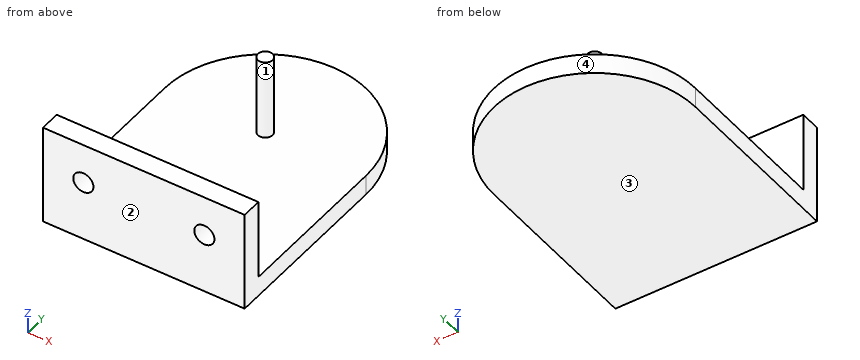
from build123d import *

# Parameters (mm, degrees)
BOSS_EXTRUDE1_DEPTH = 3.175
SKETCH4_W           = 31.75
SKETCH4_H           = 3.175
BOSS_EXTRUDE2_DEPTH = 12.7
SKETCH5_R           = 1.5875
CUT_EXTRUDE2_DEPTH  = 47.651371748
SKETCH6_R           = 1.15
BOSS_EXTRUDE3_DEPTH = 12.7


with BuildPart() as part:
    # Sketch1 → Boss-Extrude1 (new body)
    with BuildSketch(Plane.XY):
        with BuildLine():
            ThreePointArc((15.875, 0), (0, 15.875), (-15.875, 0))
            Line((-15.875, 0), (15.875, 0))
        make_face()
        with BuildLine():
            ThreePointArc((15.875, 0), (0, -15.875), (-15.875, 0))
            Line((-15.875, 0), (-15.875, -28.194))
            Line((-15.875, -28.194), (15.875, -28.194))
            Line((15.875, -28.194), (15.875, 0))
        make_face()
        with BuildLine():
            Line((15.875, 0), (-15.875, 0))
            ThreePointArc((-15.875, 0), (0, -15.875), (15.875, 0))
        make_face()
    extrude(amount=BOSS_EXTRUDE1_DEPTH)

    # Sketch4 → Boss-Extrude2 (add)
    with BuildSketch(Plane.XY.offset(3.175)):
        with Locations((0, -26.6065)):
            Rectangle(SKETCH4_W, SKETCH4_H)
    extrude(amount=BOSS_EXTRUDE2_DEPTH)

    # Sketch5 → Cut-Extrude2 (cut, through all)
    with BuildSketch(Plane(origin=(0, -25.019, 0), x_dir=(1, 0, 0), z_dir=(0, 1, 0))):
        with Locations(Location((-9.525, -9.525, 0), (0, 0, 270))):
            Circle(SKETCH5_R)
        with Locations(Location((9.525, -9.525, 0), (0, 0, 90))):
            Circle(SKETCH5_R)
    extrude(amount=-CUT_EXTRUDE2_DEPTH, mode=Mode.SUBTRACT)

    # Sketch6 → Boss-Extrude3 (add, through all)
    with BuildSketch(Plane.XY.offset(3.175)):
        Circle(SKETCH6_R)
    extrude(amount=BOSS_EXTRUDE3_DEPTH)


solid = part.part
Can you work these out from the model? Positions are in its coordinate system, mm. Face numbers are marked on the shaded views. Give positions to 0.01 mm unless a question says otherwise; leave off trailing zeros. Loops run counter-clockwise (first coordinate to the right, second up) from the corner with the lowest first, then second, coordinate; pieces in that order, holes last. Notation, with made-up numbers: (-4, 7.5) - (7, 7.5) arc R19 ccw to (7, 32.5) - close; hole circle Ø3 at (57, 18.25). An arc over 180 degrees is marked (long way). Return JSON: item names as keys, results as strings.
1. I'm going to push flat-ended pins straight in: pin 1 Ø6 at (x, y) = (-6.5, -5.5) entering from +Z (3 decimals); pin 2 Ø8 at (x, z) = (12, 1.5) entering from +Y; pin 3 Ø6 at (x, z) = (-12, 2) entering from +Y; pin 4 Ø10 at (x, y) = (6, -4.5) entering from -Z. Where does each tip first touch, or does it pass through?
Output values:
{"pin 1": "stops at z = 3.175", "pin 2": "stops at y = 13.71", "pin 3": "stops at y = 13.08", "pin 4": "stops at z = 0"}
2. If I drill on line 1 (Z direction, x = 0.5, y = 8) (3 decimals); line 2 (Y direction, x = 0.5, z = 2.25); line 3 (Y direction, x = -5, z = 11), over which ranges is the centre line in solid material (lowest first)?
Output values:
{"line 1": "z = 0 to 3.175", "line 2": "y = -28.19 to 15.87", "line 3": "y = -28.19 to -25.02"}
3. We'd pull the mould along Y, two halves only. Please class the marked faces 1, 2, 3 and 4: +Y half, -Y half, draft (parallel to the pull), parting line (faces both ways), or undercut.
Output values:
{"face 1": "undercut", "face 2": "-Y half", "face 3": "draft", "face 4": "+Y half"}
4. I want a section at D-D on z = 2.5. Please give me the cut outline in (x, y) (3 decimals), and give its area (3 significant figures).
Output values:
{"outline": "(-15.875, -28.194) - (15.875, -28.194) - (15.875, 0) arc R15.875 ccw to (-15.875, 0) - close", "area": "1,290 mm²"}
5. I want a section at A-A on z = 12. Please give me the cut outline in (x, y) (3 decimals).
Output values:
{"outline": "(-15.875, -28.194) - (15.875, -28.194) - (15.875, -25.019) - (-15.875, -25.019) - close; circle Ø2.3 at (0, 0)"}
6. I want a section at B-B on x = 0. Please give me the cut outline in (y, z) (3 decimals).
Output values:
{"outline": "(-28.194, 0) - (15.875, 0) - (15.875, 3.175) - (1.15, 3.175) - (1.15, 15.875) - (-1.15, 15.875) - (-1.15, 3.175) - (-25.019, 3.175) - (-25.019, 15.875) - (-28.194, 15.875) - close"}
7. I want a section at C-C on y = 7. Please give me the cut outline in (x, z) (3 decimals).
Output values:
{"outline": "(-14.248, 0) - (14.248, 0) - (14.248, 3.175) - (-14.248, 3.175) - close"}
